Build history of the part. All positions in model axes, mm. A direction names the side the tool comes from. Give positions to 0.01 mm unless a question says otherwise; leave off trailing zeros. Loops run counter-clockwise (first coordinate to the right, second up) from the corner with the lowest first, then second, coordinate; pieces in that order, holes last. Notation, with made-up numbers: (87.25, -29) -> (110.25, -29) arc R26 cw to (110.25, -7) -> close; hole circle Ø2 at (70.25, -21). An arc over 180 degrees is marked (long way). Answer as a JSON object with one key per item and string values. Group by question number.
Q1. Tool access for faces 5 (the flat face through (-9, 0, 4)), 6 (the flat face through (-10, 5, 3)), 7 (the cylindrical face through (-13.19, 6.82, 1.48)): list every direction of +Z, -Z, +X, -X, +Y, -Y with a clear straight run to the whole face (end or side of a thin tool).
Q2. Drop flat-ended pins along their axis: pin 1 (6.5 mm diameter, centred on x = -11.5, y = -6, fed in from +Z); pin 2 (6.5 mm diameter, centred on x = -11, y = 7.5, fed in from +Z); pin 3 (6 mm diameter, centred on x = -24.5, z = 2, fed in from +Y). Give the stop position or say it passes through.
Q3. Band-saw the part on B-B, the plane y = -17.5. Write the cut outline in (x, z), plus the area to 3 significant figures.
Q4. Two-plate mould, pull along X, no slides. Class faces 1 (the flat face through (-11, -5, 3)), 2 (the flat face through (-22, 0, 0)), 3 (the cylindrical face through (-20.52, 26.59, 3.16)), 4 (the cylindrical face through (-13.19, -6.68, 1.48)): pulls with the +X half, pulls with the -X half, needs draft (parallel to the pull), parting line crosses it, or undercut.
Q5. Band-saw the part on A-A, the plane z = 1.5. Write the cut outline in (x, y).
Q6. Band-saw the part on C-C, the plane x = -20. Write the cut outline in (y, z).
Q7. Band-saw the part on D-D, the plane y = 12. Write the cut outline in (x, z), plus the area to 3 significant figures.
Q8. Wall check: probe 1 along Y at (x, z) = (-12.5, 4); probe 2 along X at (y, z) = (6.75, 1.95); probe 3 along X at (y, z) = (-6.75, 1.45). Give the ranges that are in metal, low to high. Write a range as from..to.
from build123d import *

# Parameters (mm, degrees)
SKETCH_1_W          = 35.317292642
SKETCH_1_H          = 60
SKETCH_1_R          = 1.5
EXTRUDE_1_DEPTH     = 8
SKETCH_2_R          = 3
CUT_EXTRUDE_1_DEPTH = 3
EXTRUDE_2_DEPTH     = 60
FILLET_1_R          = 3
SKETCH_4_R          = 5
CUT_EXTRUDE_2_DEPTH = 47.960729747
CUT_EXTRUDE_3_DEPTH = 10
FILLET_2_R          = 20
CUT_EXTRUDE_4_DEPTH = 71.495063746
CUT_EXTRUDE_5_DEPTH = 2
CUT_EXTRUDE_6_DEPTH = 48.639836404
CUT_EXTRUDE_7_DEPTH = 71.495063746
FILLET_4_R          = 3


with BuildPart() as part:
    # 草图1 → 凸台-拉伸1 (new body)
    with BuildSketch(Plane.XY):
        Rectangle(SKETCH_1_W, SKETCH_1_H)
        with Locations((0, 13.5)):
            Circle(SKETCH_1_R, mode=Mode.SUBTRACT)
        with Locations((11.691342951, 6.75)):
            Circle(SKETCH_1_R, mode=Mode.SUBTRACT)
        with Locations((11.691342951, -6.75)):
            Circle(SKETCH_1_R, mode=Mode.SUBTRACT)
        with Locations((0, -13.5)):
            Circle(SKETCH_1_R, mode=Mode.SUBTRACT)
        with Locations((-11.691342951, -6.75)):
            Circle(SKETCH_1_R, mode=Mode.SUBTRACT)
        with Locations((-11.691342951, 6.75)):
            Circle(SKETCH_1_R, mode=Mode.SUBTRACT)
    extrude(amount=EXTRUDE_1_DEPTH)

    # 草图2 → 切除-拉伸1 (cut)
    with BuildSketch(Plane.XY.offset(8)):
        with Locations((0, 13.5)):
            Circle(SKETCH_2_R)
        with Locations((11.691342951, 6.75)):
            Circle(SKETCH_2_R)
        with Locations((11.691342951, -6.75)):
            Circle(SKETCH_2_R)
        with Locations((0, -13.5)):
            Circle(SKETCH_2_R)
        with Locations((-11.691342951, -6.75)):
            Circle(SKETCH_2_R)
        with Locations((-11.691342951, 6.75)):
            Circle(SKETCH_2_R)
    extrude(amount=-CUT_EXTRUDE_1_DEPTH, mode=Mode.SUBTRACT)

    # 草图3 → 凸台-拉伸2 (add)
    with BuildSketch(Plane.XZ.offset(30)):
        Polygon((-23.303511793, 11.324481191), (-17.658646321, 8), (-17.658646321, 0), (-35.232231527, 0), (-35.232231527, 11.324481191), align=None)
    extrude(amount=-EXTRUDE_2_DEPTH)

    # 圆角1
    fillet_1_edges = [part.edges().sort_by_distance(p)[0] for p in [
        (-17.658646321, 0, 8),
        (-35.232231527, 0, 11.324481191),
        (17.658646321, -30, 4),
        (-35.232231527, 0, 0),
        (-23.303511793, 0, 11.324481191),
        (17.658646321, 30, 4),
    ]]
    fillet(fillet_1_edges, radius=FILLET_1_R)

    # 草图4 → 切除-拉伸2 (cut, through all)
    with BuildSketch(Plane.XY.offset(8)):
        Circle(SKETCH_4_R)
    extrude(amount=-CUT_EXTRUDE_2_DEPTH, mode=Mode.SUBTRACT)

    # 草图5 → 切除-拉伸3 (cut)
    with BuildSketch(Plane.XY.offset(8)):
        with BuildLine():
            ThreePointArc((14.658646321, -30), (16.779966665, -29.121320344), (17.658646321, -27))
            Line((17.658646321, -27), (17.658646321, 27))
            ThreePointArc((17.658646321, 27), (16.779966665, 29.121320344), (14.658646321, 30))
            Line((14.658646321, 30), (-16.840879336, 30))
            Line((-16.840879336, 30), (-6.840879336, 10))
            Line((-6.840879336, 10), (-6.840879336, 0))
            Line((-6.840879336, 0), (-6.840879336, -10))
            Line((-6.840879336, -10), (-16.840879336, -30))
            Line((-16.840879336, -30), (14.658646321, -30))
        make_face()
    extrude(amount=-CUT_EXTRUDE_3_DEPTH, mode=Mode.SUBTRACT)

    # 圆角2
    fillet_2_edges = [part.edges().sort_by_distance(p)[0] for p in [
        (-6.840879336, -10, 4),
        (-6.840879336, 10, 4),
    ]]
    fillet(fillet_2_edges, radius=FILLET_2_R)

    # 草图6 → 切除-拉伸4 (cut, through all)
    with BuildSketch(Plane.XZ.offset(30)):
        with BuildLine():
            Line((-18.363290882, 8.414992633), (-16.840879336, 7.518385164))
            Line((-16.840879336, 7.518385164), (-16.840879336, 8))
            ThreePointArc((-16.840879336, 8), (-17.629859025, 8.105606963), (-18.363290882, 8.414992633))
        make_face()
        Polygon((-16.840879336, 8), (-16.840879336, 7.518385164), (-10.866770961, 4), (-6.840879336, 4), (-6.840879336, 8), (-8.952335516, 8), align=None)
        with BuildLine():
            Line((-28.285671321, 11.324481191), (-16.840879336, 6.512055498))
            Line((-16.840879336, 6.512055498), (-16.840879336, 7.518385164))
            Line((-16.840879336, 7.518385164), (-18.363290882, 8.414992633))
            Line((-18.363290882, 8.414992633), (-22.598867233, 10.909488557))
            ThreePointArc((-22.598867233, 10.909488557), (-23.332299089, 11.218874227), (-24.121278778, 11.324481191))
            Line((-24.121278778, 11.324481191), (-28.285671321, 11.324481191))
        make_face()
        Polygon((-16.840879336, 7.518385164), (-16.840879336, 6.512055498), (-10.866770961, 4), align=None)
    extrude(amount=-CUT_EXTRUDE_4_DEPTH, mode=Mode.SUBTRACT)

    # 草图7 → 切除-拉伸5 (cut)
    with BuildSketch(Plane.XY.offset(5)):
        with BuildLine():
            ThreePointArc((-13.244946275, 9.316382028), (-14.691342951, 6.75), (-13.244946275, 4.183617972))
            Line((-13.244946275, 4.183617972), (-13.244946275, 9.316382028))
        make_face()
        with BuildLine():
            Line((-13.244946275, 9.316382028), (-13.244946275, 4.183617972))
            ThreePointArc((-13.244946275, 4.183617972), (-10.218388433, 4.13649565), (-8.691342951, 6.75))
            ThreePointArc((-8.691342951, 6.75), (-10.218388433, 9.36350435), (-13.244946275, 9.316382028))
        make_face()
        with BuildLine():
            Line((-13.244946275, -9.316382028), (-13.244946275, -4.183617972))
            ThreePointArc((-13.244946275, -4.183617972), (-14.691342951, -6.75), (-13.244946275, -9.316382028))
        make_face()
        with BuildLine():
            ThreePointArc((-13.244946275, -4.183617972), (-14.691342951, -6.75), (-13.244946275, -9.316382028))
            Line((-13.244946275, -9.316382028), (-13.244946275, -4.183617972))
        make_face()
        with BuildLine():
            Line((-13.244946275, -4.183617972), (-13.244946275, -9.316382028))
            ThreePointArc((-13.244946275, -9.316382028), (-10.218388433, -9.36350435), (-8.691342951, -6.75))
            ThreePointArc((-8.691342951, -6.75), (-10.218388433, -4.13649565), (-13.244946275, -4.183617972))
        make_face()
    extrude(amount=-CUT_EXTRUDE_5_DEPTH, mode=Mode.SUBTRACT)

    # 草图8 → 切除-拉伸6 (cut, through all)
    with BuildSketch(Plane.XY.offset(11.324481191)):
        with BuildLine():
            ThreePointArc((-10.866770961, 18.051783249), (-18.640704436, 25.389749731), (-28.285671321, 30))
            Line((-28.285671321, 30), (-16.840879336, 30))
            Line((-16.840879336, 30), (-10.866770961, 18.051783249))
        make_face()
        with BuildLine():
            Line((-16.840879336, -30), (-10.866770961, -18.051783249))
            ThreePointArc((-10.866770961, -18.051783249), (-18.640704436, -25.389749731), (-28.285671321, -30))
            Line((-28.285671321, -30), (-16.840879336, -30))
        make_face()
    extrude(amount=-CUT_EXTRUDE_6_DEPTH, mode=Mode.SUBTRACT)

    # 草图10 → 切除-拉伸7 (cut, through all)
    with BuildSketch(Plane.XZ.offset(30)):
        with BuildLine():
            Line((-10.866770961, 4), (-28.285671321, 11.324481191))
            ThreePointArc((-28.285671321, 11.324481191), (-20.236995628, 6.090803021), (-10.866770961, 4))
        make_face()
    extrude(amount=-CUT_EXTRUDE_7_DEPTH, mode=Mode.SUBTRACT)

    # 圆角4
    fillet_4_edges = [part.edges().sort_by_distance(p)[0] for p in [
        (-28.285671321, 0, 11.324481191),
    ]]
    fillet(fillet_4_edges, radius=FILLET_4_R)


solid = part.part
Worked answers:
{
 "1": {"face 5": "+Z, +X, +Y, -Y", "face 6": "+Z", "face 7": "+Z, -Z"},
 "2": {"pin 1": "z = 4.44", "pin 2": "z = 4.32", "pin 3": "y = 29.75"},
 "3": {"outline": "(-35.23, 3) arc R3 ccw to (-32.23, 0) -> (-10.59, 0) -> (-10.59, 4) -> (-10.87, 4) arc R27.03 cw to (-27.47, 10.59) arc R3 ccw to (-29.44, 11.32) -> (-32.23, 11.32) arc R3 ccw to (-35.23, 8.32) -> close", "area": "188 mm2"},
 "4": {"face 1": "undercut", "face 2": "needs draft", "face 3": "pulls with the +X half", "face 4": "undercut"},
 "5": {"outline": "(-34.83, -30) -> (-28.29, -30) arc R34.55 ccw to (-10.87, -18.05) -> (-8.95, -14.22) arc R20 ccw to (-6.84, -5.28) -> (-6.84, 5.28) arc R20 ccw to (-8.95, 14.22) -> (-10.87, 18.05) arc R34.55 ccw to (-28.29, 30) -> (-34.83, 30) -> close; hole circle Ø3 at (-11.69, -6.75); hole circle Ø3 at (-11.69, 6.75)"},
 "6": {"outline": "(-26.28, 0) -> (26.28, 0) -> (26.28, 5.99) -> (-26.28, 5.99) -> close"},
 "7": {"outline": "(-35.23, 3) arc R3 ccw to (-32.23, 0) -> (-8, 0) -> (-8, 4) -> (-10.87, 4) arc R27.03 cw to (-27.47, 10.59) arc R3 ccw to (-29.44, 11.32) -> (-32.23, 11.32) arc R3 ccw to (-35.23, 8.32) -> close", "area": "198 mm2"},
 "8": {"probe 1": "-20.01..-9.64, -3.86..3.86, 9.64..20.01", "probe 2": "-35.04..-13.19, -10.19..-6.9", "probe 3": "-34.8..-13.19, -10.19..-6.9"}
}
